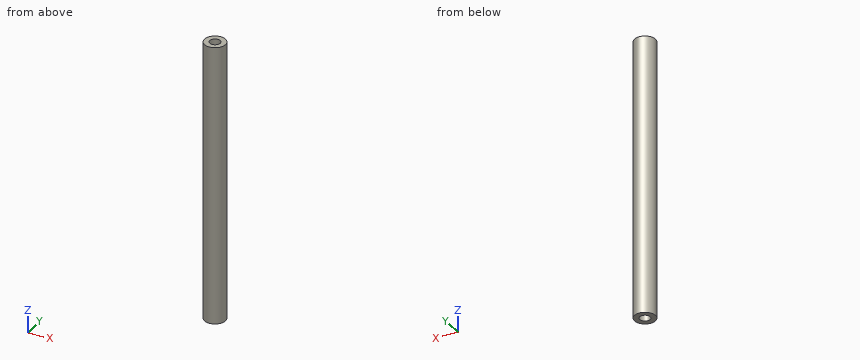
Autodesk Inventor part; units mm, degrees
ref_plane "YZ Plane" through (0, 0, 0) normal (1, 0, 0) x (0, 1, 0)
ref_plane "XZ Plane" through (0, 0, 0) normal (0, 1, 0) x (-1, 0, 0)
ref_plane "XY Plane" through (0, 0, 0) normal (0, 0, 1) x (1, 0, 0)
sketch "スケッチ1" plane through (0, 0, 0) normal (0, 0, 1) x (1, 0, 0)
  circle A0 centre (0, 0) radius 3
  circle A1 centre (0, 0) radius 1.5005
  dimension "d0" = 6
  dimension "d1" = 3.001
extrude "押し出し1" add sketch "スケッチ1" along normal blind 80
sketch "スケッチ2" plane through (0, 0, 80) normal (0, 0, 1) x (1, 0, 0)
  circle A0 centre (0, 0) radius 1.5005
  circle A1 centre (0, 0) radius 1.5
  dimension "d4" = 3
extrude "押し出し2" add sketch "スケッチ2" against normal blind 80
hole "穴1" at (0, 0, 80) direction (0, 0, -1) diameter 3 depth 6 tip angle 118
hole "穴2" at (0, 0, 0) direction (0, 0, 1) diameter 3 depth 6 tip angle 118
properties part number "スペーサーm3-80　簡易筒型" material "アルミニウム 2014-T4"
Check sheet for the modelled part. Datum: model origin and axes. Units: mm. Round coordinates to 2 decimals unless told otherwise and drop trailing zeros. Loops run counter-clockwise (first coordinate to the right, second up) from the corner with the lowest first, then second, coordinate; pieces in that order, holes last. Notation, with made-up numbers: M -26,83.25 L -11,83.25 A16 ccw -11,100.25 Z; hole C -25.75,17.5 d10. An arc over 180 degrees is marked long. One line per question, with ' | ' between items. Start each with the question number.
Item 1: Section check C-C (y = 2.25). Record the boundary of the cut face in (x, z).
Item 2: Scan lines: probe 1 along Y at (x, z) = (0, 77); probe 2 along X at (y, z) = (0.15, 58); probe 3 along Z at (x, y) = (-0.9, 0.45). Record each from-to range of solid material in increasing order.
Item 3: Section check B-B (x = 2.3). Record the boundary of the cut face in (y, z).
Item 4: Gauge pin test, flat ends, axial feed: pin 1 Ø1.5 at (x, z) = (1, 26.5) entering from -Y; pin 2 Ø1.8 at (x, y) = (0, 0) entering from -Z. Record the tip position at first contact, or that the pin passes through.
Item 5: Section check A-A (z = 48). Record the boundary of the cut face in (x, y), and give its area (3 significant figures).
Worked out:
1) outline: M -1.98,0 L 1.98,0 L 1.98,80 L -1.98,80 Z
2) probe 1: -3 to -1.5, 1.5 to 3 | probe 2: -3 to 3 | probe 3: 6.3 to 73.7
3) outline: M -1.93,0 L 1.93,0 L 1.93,80 L -1.93,80 Z
4) pin 1: y = -2.99 | pin 2: z = 6.36
5) outline: C 0,0 d6 | area: 28.3 mm^2
